Here's how the part is built. I have some questions about the finished solid (model axes, mm). A direction names the side the tool comes from. Round coordinates to 2 decimals unless told otherwise and drop trailing zeros. Answer as CSV lines item,"result".
Autodesk Inventor part; units mm, degrees
ref_plane "YZ Plane" through (0, 0, 0) normal (1, 0, 0) x (0, 1, 0)
ref_plane "XZ Plane" through (0, 0, 0) normal (0, 1, 0) x (-1, 0, 0)
ref_plane "XY Plane" through (0, 0, 0) normal (0, 0, 1) x (1, 0, 0)
sketch "Sketch1" plane through (0, 0, 0) normal (0, 0, 1) x (1, 0, 0)
  line L0 (-92.5, 40) -> (-92.5, 95)
  line L1 (-92.5, 95) -> (92.5, 95)
  line L2 (92.5, -95) -> (-92.5, -95)
  line L3 (-92.5, -95) -> (-92.5, -40)
  line L4 (-92.5, 95) -> (-62.5, 95)
  line L5 (-62.5, 40) -> (-62.5, -40)
  line L6 (92.5, 95) -> (62.5, 95)
  line L7 (62.5, -15) -> (62.5, 40)
  line L8 (-92.5, 95) -> (-92.5, 40)
  line L9 (-92.5, 40) -> (-62.5, 40)
  line L10 (-92.5, -95) -> (-92.5, -40)
  line L11 (-92.5, -40) -> (-62.5, -40)
  line L12 (62.5, 40) -> (92.5, 40)
  line L13 (62.5, -40) -> (92.5, -40)
  line L14 (92.5, 95) -> (92.5, 40)
  line L15 (92.5, -40) -> (92.5, -95)
  line L16 (-92.5, -95) -> (-77.5, -95)
  line L17 (92.5, -95) -> (77.5, -95)
  line L18 (92.5, 95) -> (77.5, 95)
  line L19 (-92.5, 95) -> (-77.5, 95)
  line L20 (62.5, -40) -> (62.5, -20)
  line L21 (-62.5, -20) -> (-62.5, -40)
  line L22 (-62.5, -20) -> (-62.5, -10)
  line L23 (-62.5, -20) -> (-62.5, -25)
  line L24 (-56.5, -29) -> (-56.5, -25)
  line L25 (-56.5, -25) -> (-47.5, -25)
  line L26 (-47.5, -25) -> (-47.5, -29)
  line L27 (6, -29) -> (6, -25)
  line L28 (15, -25) -> (15, -29)
  line L29 (-47.5, -25) -> (-56.5, -25)
  line L30 (62.5, -20) -> (62.5, -21.75)
  line L31 (62.5, -15) -> (62.5, -21.75)
  line L32 (-56.5, -25) -> (-56.5, -29)
  line L33 (-56.5, -29) -> (-47.5, -29)
  line L34 (6, -29) -> (15, -29)
  line L35 (-62.5, -15) -> (-62.5, -20)
  line L36 (6, -25) -> (15, -25)
  circle A0 centre (-77.5, 80) radius 1.5
  circle A1 centre (77.5, 80) radius 1.5
  circle A2 centre (-77.5, -80) radius 1.5
  circle A3 centre (77.5, -80) radius 1.5
  circle A4 centre (12, -85) radius 1.5
  circle A5 centre (12, -55) radius 1.5
  circle A6 centre (-12, -55) radius 1.5
  circle A7 centre (-12, -85) radius 1.5
  circle A8 centre (-38.5, -60) radius 1.5
  circle A9 centre (-24, -60) radius 1.5
  circle A10 centre (24, -60) radius 1.5
  circle A11 centre (38.5, -60) radius 1.5
  circle A12 centre (0, -15) radius 1.5
  circle A13 centre (42, 14) radius 1.5
  circle A14 centre (42, 22) radius 1.5
  circle A15 centre (-42, 22) radius 1.5
  circle A16 centre (-42, 14) radius 1.5
  circle A17 centre (-11.5, 56) radius 1.5
  circle A18 centre (11.5, 56) radius 1.5
  circle A19 centre (11.5, 85) radius 1.5
  circle A20 centre (-11.5, 85) radius 1.5
  circle A21 centre (-26.5, 54.5) radius 1
  circle A22 centre (22.5, 54.5) radius 1
  circle A23 centre (22.5, -3.5) radius 1
  circle A24 centre (-26.5, -3.5) radius 1
  point P0 (0, 0)
extrude "Extrusion1" add sketch "Sketch1" along normal blind 3
fillet "Fillet1" radius 15 4 edges at (92.5, 95, 1.5) (-92.5, 95, 1.5) (-92.5, -95, 1.5) (92.5, -95, 1.5)
fillet "Fillet2" radius 5 8 edges at (-92.5, 40, 1.5) (-62.5, 40, 1.5) (-62.5, -40, 1.5) (-92.5, -40, 1.5) (92.5, -40, 1.5) (62.5, -40, 1.5) (92.5, 40, 1.5) (62.5, 40, 1.5)
properties part number "Chassis"
1. If I drill on line 1 (Y direction, x = 42, z = 2.7); line 2 (Y direction, x = 77.5, z = 1.9); line 3 (X direction, y = -85, z = 0.85), over which ranges is the centre line in solid material (lowest first)?
Numbers:
line 1,"y = -95 to 12.5, 15.5 to 20.5, 23.5 to 95"
line 2,"y = -95 to -81.5, -78.5 to -40, 40 to 78.5, 81.5 to 95"
line 3,"x = -91.64 to -13.5, -10.5 to 10.5, 13.5 to 91.64"
2. If we mould it in two halves opening along Y, with no side actions, what happens to faces 4 (the face through (-88.22, -90.49, 1.52)), 5 (the face through (91.07, -41.5, 1.52)), 6 (the face through (63.93, -38.5, 1.52)), 7 (the face through (88.22, 90.49, 1.52))? For each: released by +Y, released by -Y, zero draft, split by the parting line, or undercut.
Numbers:
face 4,"released by -Y"
face 5,"undercut"
face 6,"undercut"
face 7,"released by +Y"
3. On a 3-axis mill with a long thin cutter (end or side, diameter ignored), from which of +Z, -Z, +X, -X, +Y, -Y can I reach the whole of each face in a straight line? I mean faces 1 (the face through (87.99, -90.72, 1.52)), 2 (the face through (64, 38.57, 1.52)), 3 (the face through (-63.93, 38.5, 1.52)). Say none if no direction works.
Numbers:
face 1,"+Z, -Z, +X, -Y"
face 2,"+Z, -Z, +X"
face 3,"+Z, -Z, -X"
4. For pin 1 Ø0.9 at (y, z) = (-1.5, 2) entering from -X, with a flat end and sliding along its axis, tell me the tip position at first contact or that it passes through.
Numbers:
pin 1,"stops at x = -62.5"
